Autodesk Inventor part; units mm, degrees
ref_plane "YZ Plane" through (0, 0, 0) normal (1, 0, 0) x (0, 1, 0)
ref_plane "XZ Plane" through (0, 0, 0) normal (0, 1, 0) x (-1, 0, 0)
ref_plane "XY Plane" through (0, 0, 0) normal (0, 0, 1) x (1, 0, 0)
sketch "Sketch4" plane through (0, 0, 0) normal (0, 0, 1) x (1, 0, 0)
  line L0 (-102.025, 0) -> (106.725, 0)
  line L1 (-28.375, 11.5) -> (15.625, 11.5)
  line L2 (15.625, 11.5) -> (15.625, 12.5)
  line L3 (15.625, 12.5) -> (60.625, 12.5)
  line L4 (60.625, 12.5) -> (60.625, 8.5)
  line L5 (60.625, 8.5) -> (89.625, 8.5)
  line L6 (89.625, 8.5) -> (89.625, 7)
  line L7 (89.625, 7) -> (106.725, 7)
  line L8 (106.725, 7) -> (106.725, 0)
  line L9 (-28.375, 11.5) -> (-28.375, 9.125)
  line L10 (-28.375, 9.125) -> (-60.625, 9.125)
  line L11 (-60.625, 9.125) -> (-60.625, 8.5)
  line L12 (-60.625, 8.5) -> (-85.125, 8.5)
  line L13 (-85.125, 8.5) -> (-85.125, 7)
  line L14 (-85.125, 7) -> (-102.025, 7)
  line L15 (-102.025, 7) -> (-102.025, 0)
  line L16 (0, 0) -> (0, 42.8251) construction
  dimension "d12" = 14
  dimension "d13" = 17
  dimension "d16" = 23
  dimension "d18" = 25
  dimension "d20" = 18.25
  dimension "d30" = 89
  dimension "d31" = 45
  dimension "d32" = 29
  dimension "d33" = 17.1
  dimension "d34" = 32.25
  dimension "d35" = 24.5
  dimension "d36" = 16.9
revolve "Revolution1" add sketch "Sketch4" angle 360 about axis through (-102.025, 0, 0) along (1, 0, 0)
chamfer "Chamfer1" distance 1 angle 45 2 edges at (106.725, -7, 0) (-102.025, -7, 0)
sketch "Sketch5" plane through (106.725, 0, 0) normal (1, 0, 0) x (0, 0, -1)
  circle A0 centre (0, 0) radius 7
  line L0 (-5, 4.899) -> (-5, -4.899)
  line L1 (5, -4.899) -> (5, 4.899)
  point P0 (0, 0)
  dimension "d27" = 10
extrude "Extrusion4" cut sketch "Sketch5" against normal up to surface (17.1 mm away) contours A0 L1 | L0 A0
ref_plane "Work Plane1" through (2.35, -3.3166, -5) normal (1, 0, 0) x (0, 0, -1)
mirror "Mirror1" about plane through (2.35, -3.3166, -5) normal (1, 0, 0) of "Extrusion4"
properties part number "axel" material "Stainless Steel"
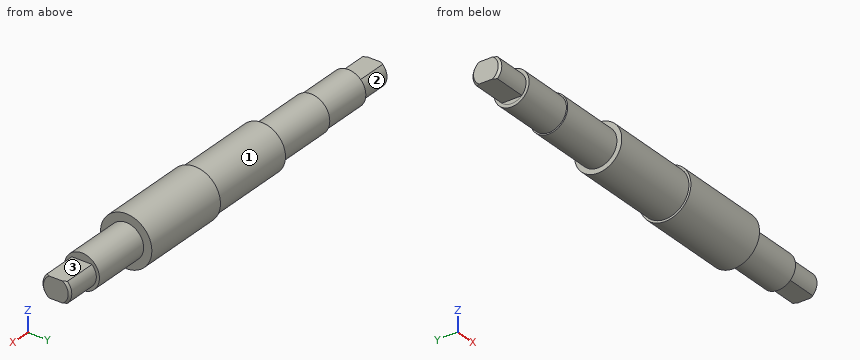
Work out the finished part from the listing and answer in its coordinate system (mm). Face numbers are marked on the shaded views. A direction names the side the tool comes from. Give positions to 0.01 mm unless a question says otherwise; leave off trailing zeros. Loops run counter-clockwise (first coordinate to the right, second up) from the corner with the lowest first, then second, coordinate; pieces in that order, holes last. Notation, with made-up numbers: (16.5, 43.25) -> (71.5, 43.25) arc R34 ccw to (71.5, 82.25) -> close; hole circle Ø11 at (-8.5, -37). An arc over 180 degrees is marked (long way). Use a Markdown table: item, result. Add a question column.
1. Section D-D on x = 11.5 is taken. Determine the outline of the cut face in (y, z).
2. For the marked faces 1, 2 and 3, determine the directions among +Z, -Z, +X, -X, +Y, -Y from which every point of the face is accessible in a straight line to the end or side of a thin tool.
3. Flat-ended cylindrical pins translate along their axes: pin 1 Ø4 at (x, y) = (-55.5, 5) entering from +Z; pin 2 Ø4 at (x, y) = (32.5, -5) entering from +Z; pin 3 Ø12 at (x, z) = (29.5, 6.5) entering from -Y. Find the tip coordinate at first contact, or state that the pin passes through.
4. Find the intervals of material crossed by probe 1 along X at (y, z) = (11, 2.5) (3 decimals); probe 2 along X at (y, z) = (-2, 6.5) (3 decimals); probe 3 along Y at (x, z) = (-58, 0.75), in increasing order.
5. Section C-C on x = -69.5 is taken. Determine the outline of the cut face in (y, z), and give its area (3 significant figures).
Results below:
| question | item | result |
|---|---|---|
| 1 | outline | circle Ø23 at (0, 0) |
| 2 | face 1 | -X |
| 2 | face 2 | -X, +Y |
| 2 | face 3 | +Z, +X, +Y, -Y |
| 3 | pin 1 | stops at z = 8.62 |
| 3 | pin 2 | stops at z = 12.13 |
| 3 | pin 3 | stops at y = -12.49 |
| 4 | probe 1 | x = -28.375 to 60.625 |
| 4 | probe 2 | x = -84.925 to 89.625 |
| 4 | probe 3 | y = -9.09 to 9.09 |
| 5 | outline | circle Ø17 at (0, 0) |
| 5 | area | 227 mm^2 |
